Autodesk Inventor part; units mm, degrees
ref_plane "YZ Plane" through (0, 0, 0) normal (1, 0, 0) x (0, 1, 0)
ref_plane "XZ Plane" through (0, 0, 0) normal (0, 1, 0) x (-1, 0, 0)
ref_plane "XY Plane" through (0, 0, 0) normal (0, 0, 1) x (1, 0, 0)
sketch "Sketch1" plane through (0, 0, 0) normal (0, 0, 1) x (1, 0, 0)
  line L0 (0, 0) -> (32.6151, 0)
  line L1 (32.6151, 0) -> (32.6151, 18.65)
  line L2 (32.6151, 18.65) -> (0, 18.65)
  line L3 (0, 18.65) -> (0, 0)
extrude "Extrusion1" add sketch "Sketch1" along normal blind 25.4
sketch "Sketch2" plane through (0, 18.65, 0) normal (0, 1, 0) x (1, 0, 0)
  line L0 (32.6151, 0) -> (32.6151, -25.4)
  line L1 (32.6151, -19.8922) -> (15.5994, -19.8922)
  line L2 (15.5994, -19.8922) -> (15.5994, -5.6439)
  line L3 (15.5994, -5.6439) -> (32.6151, -5.6439)
  line L4 (32.6151, -5.6439) -> (32.6151, -19.8922)
  line L5 (15.5994, -5.6439) -> (15.5994, -0.1361) construction
  line L6 (32.6151, -25.4) -> (0, -25.4)
  line L7 (15.5994, -25.4) -> (15.5994, -19.8922) construction
  point P0 (0, 0)
extrude "Extrusion2" cut sketch "Sketch2" against normal through all
fillet "Fillet1" radius 4.7625 2 edges at (0, 9.325, 25.4) (0, 9.325, 0)
chamfer "Chamfer1" distance 3.175 angle 45 2 edges at (32.6151, 9.325, 19.8922) (32.6151, 9.325, 5.6439)
sketch "Sketch3" plane through (15.5994, 18.65, 19.8922) normal (1, 0, 0) x (0, 0, -1)
  line L0 (14.2482, 0) -> (14.2482, -18.65)
  line L1 (14.2482, -18.65) -> (0, 0) construction
  point P0 (19.8922, -18.65)
  point P1 (7.1241, -9.325)
hole "Hole1" at (15.5994, 9.325, 12.768) direction (-1, 0, 0) diameter 3.175 end through all countersink diameter 4.7625 countersink angle 82
properties part number "Part feature intro"
Source: CAD feature listing. Evaluate the final solid. Frame: model axes, mm. A direction names the side the tool comes from. Give positions to 0.01 mm unless a question says otherwise; leave off trailing zeros. Order: outer loops, then holes, each group sorted by start corner. A loop starts at its lowest first (then second) coordinate and runs counter-clockwise, first axis right, second up. Notation, with made-up numbers: (9.25, 59.5) -> (40.25, 59.5) arc R10 cw to (40.25, 77.5) -> close; hole circle Ø11 at (19, 31). An arc over 180 degrees is marked (long way). Write item = value, one per line.
Item 1: Contact query for a flat-ended pin moving along its axis: pin 1 (3 mm diameter, centred on x = 13.5, z = 15, fed in from -Y). Output: stop coordinate, or through.
Check result:
pin_1 = 0
Item 2: Ray query, probe 1 along Z at (x, y) = (29, 3.75); probe 2 along X at (y, z) = (14.75, 19.25); probe 3 along Z at (x, y) = (30, 17.25). Return the intervals inside material, ascending.
Check result:
probe_1 = 0 to 5.64, 19.89 to 25.4
probe_2 = 0 to 15.6
probe_3 = 0 to 5.08, 20.45 to 25.4
Item 3: Section query B-B (y = 12.5). Output: boundary loops of the cut face in (x, z) (1 decimal), then the cut area to 3 significant figures.
Check result:
outline = (0, 4.8) arc R4.8 ccw to (4.8, 0) -> (32.6, 0) -> (32.6, 2.5) -> (29.4, 5.6) -> (15.6, 5.6) -> (15.6, 19.9) -> (29.4, 19.9) -> (32.6, 23.1) -> (32.6, 25.4) -> (4.8, 25.4) arc R4.8 ccw to (0, 20.6) -> close
area = 566 mm²
Item 4: Mould query, pull axis Z, two halves, no side actions, for faces 1 (the face through (1.43, 9.19, 24.04)), 2 (the face through (32.615, 9, 24)), 3 (the face through (15.599, 12, 14)). Classes: +Z half, -Z half, draft (parallel to the pull), parting line (faces both ways), or undercut.
Check result:
face_1 = +Z half
face_2 = draft
face_3 = undercut
Item 5: Section query A-A (x = 27.5). Output: boundary loops of the cut face in (y, z).
Check result:
outline = (0, 0) -> (18.65, 0) -> (18.65, 5.64) -> (0, 5.64) -> close; (0, 19.89) -> (18.65, 19.89) -> (18.65, 25.4) -> (0, 25.4) -> close
Item 6: Set-up query: faces 4 (the face through (31.005, 9.456, 4.079)), 5 (the face through (12, 0, 13)). Return all of +Z, -Z, +X, -X, +Y, -Y with unobstructed straight access to the full face (end or side cutting, diameter ignored); none if empty.
Check result:
face_4 = +X, +Y, -Y
face_5 = +Z, -Z, +X, -X, -Y
Item 7: Section query D-D (z = 18.5). Output: boundary loops of the cut face in (x, y), then the cut area to 3 significant figures.
Check result:
outline = (0, 0) -> (15.6, 0) -> (15.6, 18.65) -> (0, 18.65) -> close
area = 291 mm²
